Build history of the part. All positions in model axes, mm. Round coordinates to 2 decimals unless told otherwise and drop trailing zeros. Loops run counter-clockwise (first coordinate to the right, second up) from the corner with the lowest first, then second, coordinate; pieces in that order, holes last. Notation, with made-up numbers: (71.25, 44) - (104.25, 44) arc R19 cw to (104.25, 49) - close; hole circle Ø7 at (44.25, 9.25). An arc over 180 degrees is marked (long way). Use a Markdown table: item, result.
from build123d import *

# Parameters (mm, degrees)
SKETCH_1_R          = 2.5
EXTRUDE_1_DEPTH     = 6
CUT_EXTRUDE_1_DEPTH = 7.0000001
HOLE_WIZARD_M41_D   = 4.5
CUT_EXTRUDE_2_DEPTH = 7.0000001
FILLET_1_R          = 2
SKETCH_9_R          = 3
SKETCH_9_R_2        = 4.5
CUT_EXTRUDE_4_DEPTH = 7.0000001
FILLET_4_R          = 2
FILLET_5_R          = 10


with BuildPart() as part:
    # Эскиз1 → Бобышка-Вытянуть1 (new body)
    with BuildSketch(Plane.XY):
        with BuildLine():
            Line((6.5, -18.132817334), (6.5, -210))
            add(Edge.make_bspline(
                [(7.75, -241.602885683), (-7.119806504, -226.33675702), (6.5, -210)],
                knots=[0, 0, 0, 1, 1, 1], degree=2))
            ThreePointArc((7.75, -241.602885683), (9.397114317, -247.75), (3.25, -249.397114317))
            ThreePointArc((3.25, -249.397114317), (-6.419807766, -240.569690394), (-10, -227.975611669))
            Line((-10, -227.975611669), (-10, 0))
            ThreePointArc((-10, 0), (1.006528746, 9.949216044), (9.797379977, -2.002834391))
            Line((9.797379977, -2.002834391), (6.5, -18.132817334))
        make_face()
        with Locations((5.5, -245.5)):
            Circle(SKETCH_1_R, mode=Mode.SUBTRACT)
    extrude(amount=EXTRUDE_1_DEPTH)

    # Эскиз2 → Вырез-Вытянуть1 (cut, through all)
    with BuildSketch(Plane.XY.offset(6)):
        with BuildLine():
            Line((6.5, -198.230414456), (6.5, -191.159346644))
            ThreePointArc((6.5, -191.159346644), (-2.545169709, -194.568344894), (-0.718217458, -204.060373635))
            ThreePointArc((-0.718217458, -204.060373635), (2.797841421, -203.689793061), (2.427260847, -200.173734182))
            ThreePointArc((2.427260847, -200.173734182), (2.923396053, -195.974106866), (6.5, -198.230414456))
        make_face()
    extrude(amount=-CUT_EXTRUDE_1_DEPTH, mode=Mode.SUBTRACT)

    # Отверстие с зазором M41 (through all)
    with Locations(Plane.XY.offset(6)):
        with Locations((0, 0)):
            Hole(HOLE_WIZARD_M41_D / 2)

    # Эскиз6 → Вырез-Вытянуть2 (cut, through all)
    with BuildSketch(Plane.XY.offset(6)):
        with BuildLine():
            ThreePointArc((5.656854249, -5.656854249), (0, 8), (-5.656854249, -5.656854249))
            ThreePointArc((-5.656854249, -5.656854249), (-5.656854249, -8.485281374), (-8.485281374, -8.485281374))
            ThreePointArc((-8.485281374, -8.485281374), (0, 12), (8.485281374, -8.485281374))
            ThreePointArc((8.485281374, -8.485281374), (5.656854249, -8.485281374), (5.656854249, -5.656854249))
        make_face()
    extrude(amount=-CUT_EXTRUDE_2_DEPTH, mode=Mode.SUBTRACT)

    # Скругление1
    fillet_1_edges = [part.edges().sort_by_distance(p)[0] for p in [
        (8.468890039, -8.501484892, 3),
        (-10, -6.633249581, 3),
    ]]
    fillet(fillet_1_edges, radius=FILLET_1_R)

    # Эскиз9 → Вырез-Вытянуть4 (cut, through all)
    with BuildSketch(Plane.XY.offset(6)):
        with Locations((1, -22.672779762)):
            Circle(SKETCH_9_R)
        with Locations((1, -42.672779762)):
            Circle(SKETCH_9_R)
        with Locations((1, -62.672779762)):
            Circle(SKETCH_9_R)
        with Locations((1, -82.672779762)):
            Circle(SKETCH_9_R)
        with Locations((1, -102.672779762)):
            Circle(SKETCH_9_R)
        with Locations((1, -122.672779762)):
            Circle(SKETCH_9_R)
        with Locations((1, -142.672779762)):
            Circle(SKETCH_9_R)
        with Locations((1, -162.672779762)):
            Circle(SKETCH_9_R)
        with Locations((1, -182.672779762)):
            Circle(SKETCH_9_R)
        with Locations((-3.5, -32.672779762)):
            Circle(SKETCH_9_R_2)
        with Locations((-3.5, -52.672779762)):
            Circle(SKETCH_9_R_2)
        with Locations((-3.5, -72.672779762)):
            Circle(SKETCH_9_R_2)
        with Locations((-3.5, -92.672779762)):
            Circle(SKETCH_9_R_2)
        with Locations((-3.5, -112.672779762)):
            Circle(SKETCH_9_R_2)
        with Locations((-3.5, -132.672779762)):
            Circle(SKETCH_9_R_2)
        with Locations((-3.5, -152.672779762)):
            Circle(SKETCH_9_R_2)
        with Locations((-3.5, -172.672779762)):
            Circle(SKETCH_9_R_2)
    extrude(amount=-CUT_EXTRUDE_4_DEPTH, mode=Mode.SUBTRACT)

    # Скругление4
    fillet_4_edges = [part.edges().sort_by_distance(p)[0] for p in [
        (6.5, -191.159346644, 3),
    ]]
    fillet(fillet_4_edges, radius=FILLET_4_R)

    # Скругление5
    fillet_5_edges = [part.edges().sort_by_distance(p)[0] for p in [
        (6.5, -210, 3),
    ]]
    fillet(fillet_5_edges, radius=FILLET_5_R)


solid = part.part
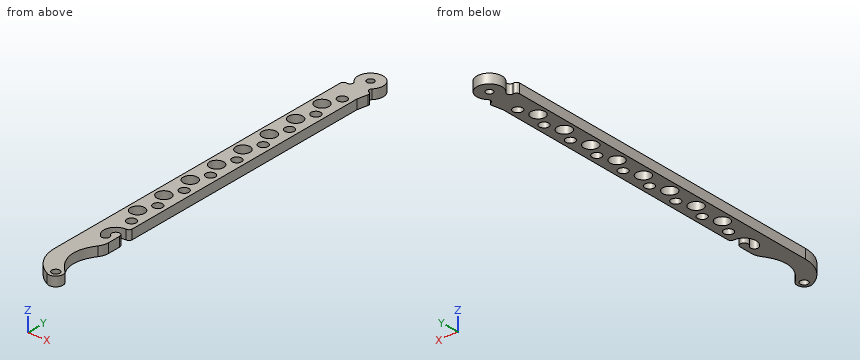
Q1. Probe line 1 (X direction, y = -62.5, z = 1); line 2 (X direction, y = -67, z = 5.25); line 3 (X direction, y = -72, z = 1.75). List the from-to ranges inside material, lowest first.
Results found:
| item | result |
|---|---|
| line 1 | x = -10 to -2, 4 to 6.5 |
| line 2 | x = -10 to 6.5 |
| line 3 | x = -10 to -7.95, 0.95 to 6.5 |
Q2. Cut at B-B, the plane z = 2.75. Count the separate pieces of the cut face and the enclosed holes in it, plus the area to 3 significant figures.
Results found:
| item | result |
|---|---|
| separate pieces | 1 |
| enclosed holes | 19 |
| area | 3,120 mm2 |
Q3. Drop flat-ended pins along their axis: pin 1 (4.5 mm diameter, centred on x = 5.5, y = -245.5, fed in from +Z); pin 2 (1.8 mm diameter, centred on y = -204.5, z = 2, fed in from +X); pin 3 (1 mm diameter, centred on x = -8, z = 1.5, fed in from -Y); pin 4 (1 mm diameter, centred on x = 2.5, z = 3, fed in from -Y). Give the stop position or say it passes through.
Results found:
| item | result |
|---|---|
| pin 1 | passes through |
| pin 2 | stops at x = 6.5 |
| pin 3 | stops at y = -238.63 |
| pin 4 | stops at y = -249.27 |
Q4. Cut at C-C, the plane y = -245.5. List the corners of the cut face in (x, z), plus the area to 3 significant figures.
Results found:
| item | result |
|---|---|
| outline | (-2.37, 0) - (3, 0) - (3, 6) - (-2.37, 6) - close; (8, 0) - (10, 0) - (10, 6) - (8, 6) - close |
| area | 44.2 mm2 |
Q5. Cut at A-A, the plane y = 0. List the corners of the cut face in (x, z).
Results found:
| item | result |
|---|---|
| outline | (-8, 0) - (-2.25, 0) - (-2.25, 6) - (-8, 6) - close; (2.25, 0) - (8, 0) - (8, 6) - (2.25, 6) - close |
